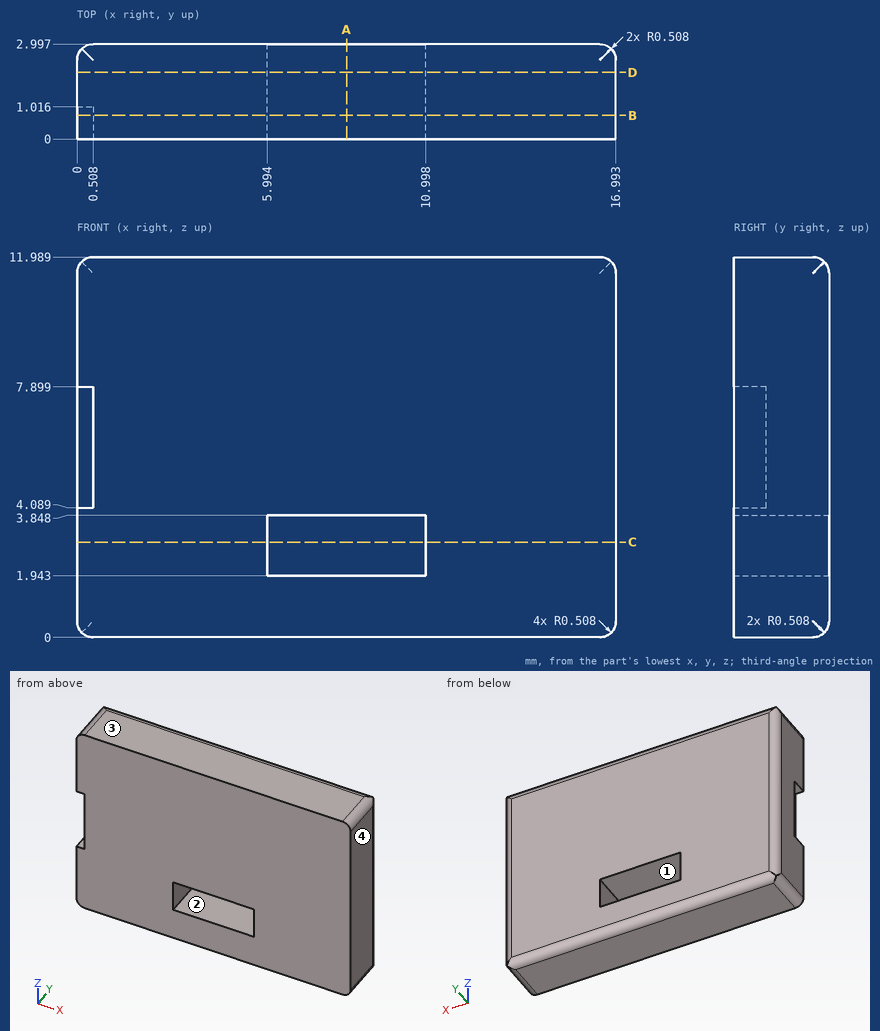
For this review, use the dimensioned drawing (mm, ordinates from the lowest corner) and the shaded views. Coordinates: 2 decimals unless noted, no trailing zeros. Loops run counter-clockwise (first coordinate to the right, second up) from the corner with the lowest first, then second, coordinate; pieces in that order, holes last.
1. Add section B-B, the plane y = 0.75. Give the boundary of the cut face in (x, z) (1 decimal), then the cut area to 3 significant figures.
2. For line 1 (Z direction, x = 10, y = 1.25); line 2 (X direction, y = 0.75, z = 3.5) (1 decimal); line 3 (Z direction, x = 4.5, y = 2.85), list the stretches that pass through material, from the lowest coordinate up.
3. Add section C-C, the plane z = 3. Give the boundary of the cut face in (x, y) (1 decimal).
4. Insertion check: P1, Ø3, axis at x = 5.5, z = 3, coming from the -Y side; P2, Ø0.8, axis at y = 0.5, z = 6.5, coming from the -X side. Each pin has a flat end and moves straight along its axis. Give the tip position at first contact, or say it passes through.
5. Mouldability with a two-part tool opening along X and no side actions: class the marked faces 1, 2, 3 and 4 as +X half, -X half, draft (parallel to the pull), parting line (faces both ways), or undercut.
6. Add section D-D, the plane y = 2.1. Give the boundary of the cut face in (x, z) (1 decimal), then the cut area to 3 significant figures.
7. Add section A-A, the plane x = 8.5. Give the boundary of the cut face in (y, z), then the cut area to 3 significant figures.
Result:
1. outline: (0, 0.5) arc R0.5 ccw to (0.5, 0) - (16.5, 0) arc R0.5 ccw to (17, 0.5) - (17, 11.5) arc R0.5 ccw to (16.5, 12) - (0.5, 12) arc R0.5 ccw to (0, 11.5) - (0, 7.9) - (0.5, 7.9) - (0.5, 4.1) - (0, 4.1) - close; hole (6, 1.9) - (11, 1.9) - (11, 3.8) - (6, 3.8) - close
1. area: 192 mm2
2. line 1: z = 0 to 1.94, 3.85 to 11.99
2. line 2: x = 0 to 6, 11 to 17
2. line 3: z = 0.15 to 11.84
3. outline: (0, 0) - (6, 0) - (6, 3) - (0.5, 3) arc R0.5 ccw to (0, 2.5) - close; (11, 0) - (17, 0) - (17, 2.5) arc R0.5 ccw to (16.5, 3) - (11, 3) - close
4. P1: stops at y = 0
4. P2: stops at x = 0.51
5. face 1: undercut
5. face 2: undercut
5. face 3: draft
5. face 4: +X half
6. outline: (0, 0.5) arc R0.5 ccw to (0.5, 0) - (16.5, 0) arc R0.5 ccw to (17, 0.5) - (17, 11.5) arc R0.5 ccw to (16.5, 12) - (0.5, 12) arc R0.5 ccw to (0, 11.5) - close; hole (6, 1.9) - (11, 1.9) - (11, 3.8) - (6, 3.8) - close
6. area: 194 mm2
7. outline: (0, 0) - (2.49, 0) arc R0.51 ccw to (3, 0.51) - (3, 1.94) - (0, 1.94) - close; (0, 3.85) - (3, 3.85) - (3, 11.48) arc R0.51 ccw to (2.49, 11.99) - (0, 11.99) - close
7. area: 30.1 mm2
